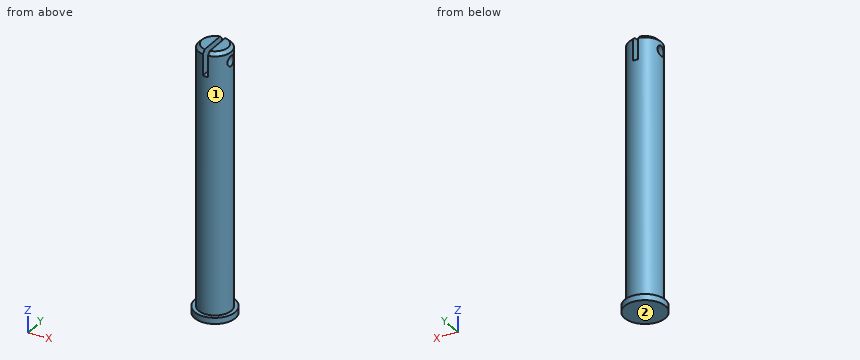
```python
from build123d import *

# Parameters (mm, degrees)
F0_R          = 31.75
F1_DEPTH      = 9.525
F2_R          = 25.4
F3_DEPTH      = 406.4
F5_DEPTH      = 38.1
F6_R          = 7.9375
F7_DEPTH      = 25.4
F7_DEPTH_BACK = 50.8
F8_SIZE       = 5.08


with BuildPart() as f1:
    # F0 (on Top) → F1 (new body)
    with BuildSketch(Plane.XY):
        Circle(F0_R)
    extrude(amount=F1_DEPTH)

    # F2 (on face) → F3 (join)
    with BuildSketch(Plane.XY.offset(9.525)):
        Circle(F2_R)
    extrude(amount=F3_DEPTH)

    # F4 (on face) → F5 (cut)
    with BuildSketch(Plane.XY.offset(415.925)):
        with BuildLine():
            ThreePointArc((3.96875, 25.088025499), (0, 25.4), (-3.96875, 25.088025499))
            Line((-3.96875, 25.088025499), (-3.96875, -25.088025499))
            ThreePointArc((-3.96875, -25.088025499), (0, -25.4), (3.96875, -25.088025499))
            Line((3.96875, -25.088025499), (3.96875, 25.088025499))
        make_face()
    extrude(amount=-F5_DEPTH, mode=Mode.SUBTRACT)

    # F6 (on face) → F7 (cut, two sides)
    with BuildSketch(Plane.YZ.offset(-3.96875)) as f7_sk:
        with Locations((0, 396.875)):
            Circle(F6_R)
    extrude(amount=-F7_DEPTH, mode=Mode.SUBTRACT)
    extrude(f7_sk.sketch, amount=F7_DEPTH_BACK, mode=Mode.SUBTRACT)

    # F8
    f8_edges = [f1.edges().sort_by_distance(p)[0] for p in [
        (-25.4, 0, 415.925),
        (19.312771, -16.497784, 415.925),
        (19.312771, 16.497784, 415.925),
    ]]
    chamfer(f8_edges, length=F8_SIZE)


solid = f1.part
```
Can you work these out from the model? Positions are in its coordinate system, mm. Face numbers are marked on the shaded views. A direction names the side the tool comes from. Round coordinates to 2 decimals unless told otherwise and drop trailing zeros. Loops run counter-clockwise (first coordinate to the right, second up) from the corner with the lowest first, then second, coordinate; pieces in that order, holes last. Notation, with made-up numbers: (25.25, 73.25) -> (60.25, 73.25) arc R26 cw to (60.25, 92.25) -> close; hole circle Ø6 at (12.25, 4). An arc over 180 degrees is marked (long way). One line per item, written item: value. Start each with the question number.
1. For pin 1 (2 mm diameter, centred on x = 18, z = 323, fed in from -Y); pin 2 (12 mm diameter, centred on x = -11.5, z = 212, fed in from -Y); pin 3 (19 mm diameter, centred on y = 11, z = 390, fed in from -X), each with a flat end and sliding along its axis, tell me the tip position at first contact or that it passes through.
2. If we section it at B-B, the plane x = 0: Write out the boundary of the cut face in (y, z) (3 decimals), then the cut area to 3 significant figures.
3. If we section it at A-A, the plane y = 0: Give the number of separate pieces and of enclosed holes in the cut face, then the cut area to 3 significant figures.
4. If we section it at C-C, the plane z = 103: Write out the boundary of the cut face in (x, y), then the cut area to 3 significant figures.
5. For the marked faces 1 and 2, which set-ups out of +Z, -Z, +X, -X, +Y, -Y let a thin tool reach every point of the face, with its end or its side?
6. If I drill on probe 1 along Z at (x, y) = (-11.25, 0) (1 decimal); probe 2 along Z at (x, y) = (8.5, -26) (3 decimals); probe 3 along Y at (x, z) = (-4, 291.5), over which ranges is the centre line in solid material (lowest first)?
Calculated:
1. pin 1: stops at y = -18.87
1. pin 2: stops at y = -24.8
1. pin 3: stops at x = -25.35
2. outline: (-31.75, 0) -> (31.75, 0) -> (31.75, 9.525) -> (25.4, 9.525) -> (25.4, 377.825) -> (-25.4, 377.825) -> (-25.4, 9.525) -> (-31.75, 9.525) -> close
2. area: 19,300 mm²
3. separate pieces: 3
3. enclosed holes: 0
3. area: 20,200 mm²
4. outline: circle Ø50.8 at (0, 0)
4. area: 2,030 mm²
5. face 1: +Z
5. face 2: -Z, +X, -X, +Y, -Y
6. probe 1: z = 0 to 388.9, 404.8 to 415.9
6. probe 2: z = 0 to 9.525
6. probe 3: y = -25.08 to 25.08
